Work out the finished part from the listing and answer in its coordinate system (mm). A direction names the side the tool comes from. Coordinates: 2 decimals unless noted, no trailing zeros. Write each loop counter-clockwise with the first axis right and the second up, starting at its lowest first coordinate (ties: lowest second). Pieces come first, ordered by that corner, then holes. Notation, with made-up numbers: (72.5, 53.5) - (127.5, 53.5) arc R11 ccw to (127.5, 66.5) - close; hole circle Ø9 at (13.5, 4.5). An arc over 180 degrees is marked (long way). Answer as a JSON object with one key per item and string values. Group by question number.
from build123d import *

# Parameters (mm, degrees)
BOSS_EXTRUDE1_DEPTH = 2
BOSS_EXTRUDE3_DEPTH = 7
FILLET5_R           = 1


with BuildPart() as part:
    # Sketch1 → Boss-Extrude1 (new body)
    with BuildSketch(Plane(origin=(0, 0, 0), x_dir=(1, 0, 0), z_dir=(0, 1, 0))):
        Polygon((4.1, -4.1), (4.1, -13.2), (-4.1, -13.2), (-4.1, -4.1), (-12.2, -4.1), (-12.2, 4.1), (-4.1, 4.1), (-4.1, 13.2), (4.1, 13.2), (4.1, 4.1), (12.2, 4.1), (12.2, -4.1), align=None)
    extrude(amount=BOSS_EXTRUDE1_DEPTH)

    # Sketch4 → Boss-Extrude3 (add)
    with BuildSketch(Plane(origin=(0, 2, 0), x_dir=(1, 0, 0), z_dir=(0, 1, 0))):
        Polygon((10.7, -2.6), (5.5, -2.6), (2.6, -2.6), (2.6, -10.7), (-2.6, -10.7), (-2.6, -2.6), (-10.7, -2.6), (-10.7, 2.6), (-5.5, 2.6), (-2.6, 2.6), (-2.6, 10.7), (2.6, 10.7), (2.6, 2.6), (5.5, 2.6), (10.7, 2.6), align=None)
    extrude(amount=BOSS_EXTRUDE3_DEPTH)

    # Fillet5
    fillet5_edges = [part.edges().sort_by_distance(p)[0] for p in [
        (6.65, 9, -2.6),
        (2.6, 9, -6.65),
        (0, 9, -10.7),
        (-2.6, 9, -6.65),
        (-6.65, 9, -2.6),
        (-10.7, 9, 0),
        (-6.65, 9, 2.6),
        (-2.6, 9, 6.65),
        (0, 9, 10.7),
        (2.6, 9, 6.65),
        (6.65, 9, 2.6),
        (10.7, 9, 0),
    ]]
    fillet(fillet5_edges, radius=FILLET5_R)


solid = part.part
Q1. Section C-C on x = -9.25 is taken. Determine the outline of the cut face in (y, z), plus the area to 3 significant figures.
Q2. Section D-D on y = 0.5 is taken. Determine the outline of the cut face in (x, z).
Q3. Flat-ended cylindrical pins translate along their axes: pin 1 Ø5 at (x, z) = (0, -6) entering from -Y; pin 2 Ø2 at (y, z) = (4, 8) entering from +X; pin 3 Ø3 at (y, z) = (4, -5.5) entering from -X; pin 4 Ø5 at (x, y) = (5, 5.5) entering from -Z. Find the tip coordinate at first contact, or state that the pin passes through.
Q4. A tool of negligible diameter and unlimited length cuts with its end or side. For faces 1 (the face through (-8, 1, -4.1)), 2 (the face through (0, 5, -10.7)), 3 (the face through (0, 5, 10.7)), 4 (the face through (-2.315, 8.699, -6.214)), from which of +Z, -Z, +X, -X, +Y, -Y can it reach the whole face along a straight path? Write none if from no direction.
Q5. Consider L1, parallel to X at y = 2.5, z = 3.25; L2, parallel to Z at x = -2, y = 2.5. Determine where each line is inside the solid, lowest interval first. Write a range as from..to.
Q6. Section A-A on y = 4.75 is taken. Determine the outline of the cut face in (x, z).
Q7. Section B-B on z = -7.25 is taken. Determine the outline of the cut face in (x, y), plus the area to 3 significant figures.
Numbers:
{
 "1": {"outline": "(0, -4.1) - (2, -4.1) - (2, -2.6) - (8, -2.6) arc R1 ccw to (9, -1.6) - (9, 1.6) arc R1 ccw to (8, 2.6) - (2, 2.6) - (2, 4.1) - (0, 4.1) - close", "area": "52.4 mm²"},
 "2": {"outline": "(-12.2, -4.1) - (-4.1, -4.1) - (-4.1, -13.2) - (4.1, -13.2) - (4.1, -4.1) - (12.2, -4.1) - (12.2, 4.1) - (4.1, 4.1) - (4.1, 13.2) - (-4.1, 13.2) - (-4.1, 4.1) - (-12.2, 4.1) - close"},
 "3": {"pin 1": "stops at y = 0", "pin 2": "stops at x = 2.6", "pin 3": "stops at x = -2.6", "pin 4": "stops at z = -10.7"},
 "4": {"face 1": "-Z, -X, +Y, -Y", "face 2": "-Z, +X, -X, +Y", "face 3": "+Z, +X, -X, +Y", "face 4": "-Z, -X, +Y"},
 "5": {"L1": "x = -2.6..2.6", "L2": "z = -10.7..10.7"},
 "6": {"outline": "(-10.7, -2.6) - (-2.6, -2.6) - (-2.6, -10.7) - (2.6, -10.7) - (2.6, -2.6) - (10.7, -2.6) - (10.7, 2.6) - (2.6, 2.6) - (2.6, 10.7) - (-2.6, 10.7) - (-2.6, 2.6) - (-10.7, 2.6) - close"},
 "7": {"outline": "(-4.1, 0) - (4.1, 0) - (4.1, 2) - (2.6, 2) - (2.6, 8) arc R1 ccw to (1.6, 9) - (-1.6, 9) arc R1 ccw to (-2.6, 8) - (-2.6, 2) - (-4.1, 2) - close", "area": "52.4 mm²"}
}
